```python
from build123d import *

# Parameters (mm, degrees)
ESBO_O1_R                = 5
ESBO_O1_R_2              = 1.65
RESSALTO_EXTRUS_O1_DEPTH = 3
FILETE1_R                = 20


with BuildPart() as part:
    # Esboço1 → Ressalto-extrusão1 (new body)
    with BuildSketch(Plane.XY):
        with BuildLine():
            Line((7.483314774, -5), (72.516685226, -5))
            ThreePointArc((72.516685226, -5), (89, 0), (72.516685226, 5))
            Line((72.516685226, 5), (7.483314774, 5))
            ThreePointArc((7.483314774, 5), (-9, 0), (7.483314774, -5))
        make_face()
        Circle(ESBO_O1_R, mode=Mode.SUBTRACT)
        with Locations((32.5, 0)):
            Circle(ESBO_O1_R_2, mode=Mode.SUBTRACT)
        with Locations((47.5, 0)):
            Circle(ESBO_O1_R_2, mode=Mode.SUBTRACT)
        with Locations((80, 0)):
            Circle(ESBO_O1_R, mode=Mode.SUBTRACT)
    extrude(amount=RESSALTO_EXTRUS_O1_DEPTH)

    # Filete1
    filete1_edges = [part.edges().sort_by_distance(p)[0] for p in [
        (72.516685226, -5, 1.5),
        (7.483314774, -5, 1.5),
        (7.483314774, 5, 1.5),
        (72.516685226, 5, 1.5),
    ]]
    fillet(filete1_edges, radius=FILETE1_R)


solid = part.part
```
Build history of the part. All positions in model axes, mm. A direction names the side the tool comes from. Give positions to 0.01 mm unless a question says otherwise; leave off trailing zeros. Order: outer loops, then holes, each group sorted by start corner. A loop starts at its lowest first (then second) coordinate and runs counter-clockwise, first axis right, second up. Notation, with made-up numbers: M 47.25,70.5 L 100.25,70.5 A35 ccw 100.25,106.5 Z; hole C 78,35 d1. An arc over 180 degrees is marked long. Write item = value, one per line. Start each with the question number.
(1) Slice it at B-B on y = 0. Write the cut outline in (x, z), plus the area to 3 significant figures.
(2) Two-plate mould, pull along X, no slides. Class faces 4 (the flat face through (39, 0, 3)), 5 (the cylindrical face through (9.52, -5.68, 1.52)): released by +X, released by -X, zero draft, split by the parting line, or undercut.
(3) Which spindle directions (+Z, -Z, +X, -X, +Y, -Y) get a long thin tool onto all of the face, cutting with end or side? Do faces 1 (the cylindrical face through (70.48, -5.68, 1.52)), 2 (the cylindrical face through (70.627, 5.722, 1.521)), 3 (the cylindrical face through (89, 0, 1)). Say none if no direction does.
(4) Slice it at A-A on x = 0. Write the cut outline in (y, z).
(5) Pin check, flat tips, straight feed: pin 1 Ø6 at (x, y) = (0, 0) entering from +Z; pin 2 Ø1.5 at (y, z) = (6.5, 1.5) entering from +X; pin 3 Ø0.9 at (x, z) = (52, 1.5) entering from +Y; pin 4 Ø1 at (y, z) = (-1.5, 0.5) entering from -X. Stop position of each tip, or through.
(6) Probe L1, parallel to Y at x = 47.5, z = 1.3; L2, parallel to X at y = 1.5, z = 1.5; L3, parallel to X at y = -2.5, z = 0.45. List the from-to ranges inside material, lowest first. Write a range as [from, to].
(7) Slice it at D-D on x = 47.5. Write the cut outline in (y, z).
(8) Slice it at C-C on z = 1.75. Write the cut outline in (x, y).
Responses:
q1.outline = M -9,0 L -5,0 L -5,3 L -9,3 Z; M 5,0 L 30.85,0 L 30.85,3 L 5,3 Z; M 34.15,0 L 45.85,0 L 45.85,3 L 34.15,3 Z; M 49.15,0 L 75,0 L 75,3 L 49.15,3 Z; M 85,0 L 89,0 L 89,3 L 85,3 Z
q1.area = 214 mm2
q2.face_4 = zero draft
q2.face_5 = undercut
q3.face_1 = +Z, -Z, -Y
q3.face_2 = +Z, -Z, +Y
q3.face_3 = +Z, -Z
q4.outline = M -9,0 L -5,0 L -5,3 L -9,3 Z; M 5,0 L 9,0 L 9,3 L 5,3 Z
q5.pin_1 = through
q5.pin_2 = 86.92
q5.pin_3 = 5
q5.pin_4 = -8.94
q6.L1 = [-5, -1.65], [1.65, 5]
q6.L2 = [-8.87, -4.77], [4.77, 31.81], [33.19, 46.81], [48.19, 75.23], [84.77, 88.87]
q6.L3 = [-8.65, -4.33], [4.33, 75.67], [84.33, 88.65]
q7.outline = M -5,0 L -1.65,0 L -1.65,3 L -5,3 Z; M 1.65,0 L 5,0 L 5,3 L 1.65,3 Z
q8.outline = M 4.56,-7.76 A20 cw 14.7,-5 L 65.3,-5 A20 cw 75.44,-7.76 A9 ccw long 75.44,7.76 A20 cw 65.3,5 L 14.7,5 A20 cw 4.56,7.76 A9 ccw long Z; hole C 0,0 d10; hole C 32.5,0 d3.3; hole C 47.5,0 d3.3; hole C 80,0 d10
